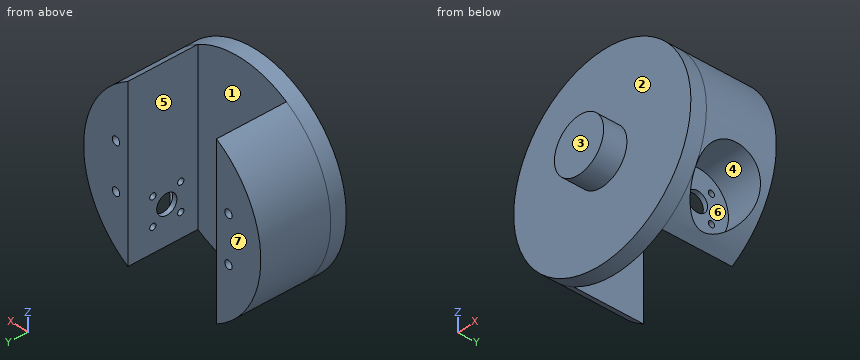
```python
from build123d import *

# Parameters (mm, degrees)
SKETCH1_R           = 17.5
BOSS_EXTRUDE1_DEPTH = 15
SKETCH2_R           = 63
BOSS_EXTRUDE2_DEPTH = 10
BOSS_EXTRUDE3_DEPTH = 45
SKETCH5_R           = 2.625
CUT_EXTRUDE1_DEPTH  = 6
SKETCH7_R           = 20
CUT_EXTRUDE2_DEPTH  = 28.5
SKETCH9_R           = 2
SKETCH9_R_2         = 6.5
CUT_EXTRUDE3_DEPTH  = 31.5


with BuildPart() as part:
    # Sketch1 → Boss-Extrude1 (new body)
    with BuildSketch(Plane(origin=(0, 0, 0), x_dir=(1, 0, 0), z_dir=(0, 1, 0))):
        with Locations(Location((0, 0, 0), (0, 0, 270))):
            Circle(SKETCH1_R)
    extrude(amount=BOSS_EXTRUDE1_DEPTH)

    # Sketch2 → Boss-Extrude2 (add)
    with BuildSketch(Plane(origin=(0, 15, 0), x_dir=(1, 0, 0), z_dir=(0, 1, 0))):
        with Locations(Location((0, 0, 0), (0, 0, 270))):
            Circle(SKETCH2_R)
    extrude(amount=BOSS_EXTRUDE2_DEPTH)

    # Sketch4 → Boss-Extrude3 (add)
    with BuildSketch(Plane(origin=(0, 25, 0), x_dir=(1, 0, 0), z_dir=(0, 1, 0))):
        with BuildLine():
            Line((-31.5, 44), (-31.5, 54.559600438))
            ThreePointArc((-31.5, 54.559600438), (-63, 0), (-31.5, -54.559600438))
            Line((-31.5, -54.559600438), (-31.5, -44))
            Line((-31.5, -44), (-31.5, 44))
        make_face()
        with BuildLine():
            Line((31.5, -44), (31.5, 44))
            Line((31.5, 44), (31.5, 54.559600438))
            ThreePointArc((31.5, 54.559600438), (63, 0), (31.5, -54.559600438))
            Line((31.5, -54.559600438), (31.5, -44))
        make_face()
    extrude(amount=BOSS_EXTRUDE3_DEPTH)

    # Sketch5 → Cut-Extrude1 (cut)
    with BuildSketch(Plane(origin=(0, 70, 0), x_dir=(1, 0, 0), z_dir=(0, 1, 0))):
        with Locations(Location((-40, 15, 0), (0, 0, 270))):
            Circle(SKETCH5_R)
        with Locations(Location((-40, -15, 0), (0, 0, 270))):
            Circle(SKETCH5_R)
        with Locations(Location((40, -15, 0), (0, 0, 90))):
            Circle(SKETCH5_R)
        with Locations(Location((40, 15, 0), (0, 0, 90))):
            Circle(SKETCH5_R)
    extrude(amount=-CUT_EXTRUDE1_DEPTH, mode=Mode.SUBTRACT)

    # Sketch7 → Cut-Extrude2 (cut)
    with BuildSketch(Plane(origin=(63, 0, 0), x_dir=(0, 0, -1), z_dir=(1, 0, 0))):
        with Locations((30, 45)):
            Circle(SKETCH7_R)
    extrude(amount=-CUT_EXTRUDE2_DEPTH, mode=Mode.SUBTRACT)

    # Sketch9 → Cut-Extrude3 (cut)
    with BuildSketch(Plane(origin=(63, 0, 0), x_dir=(0, 0, -1), z_dir=(1, 0, 0))):
        with Locations((21.019743879, 36.019743879)):
            Circle(SKETCH9_R)
        with Locations((21.019743879, 53.980256121)):
            Circle(SKETCH9_R)
        with Locations((38.980256121, 53.980256121)):
            Circle(SKETCH9_R)
        with Locations((38.980256121, 36.019743879)):
            Circle(SKETCH9_R)
        with Locations((30, 45)):
            Circle(SKETCH9_R_2)
    extrude(amount=-CUT_EXTRUDE3_DEPTH, mode=Mode.SUBTRACT)


solid = part.part
```
For this review, take the finished solid that the model builds, in its own axes (mm). Face numbers are marked on the shaded views. A direction names the side the tool comes from. Round coordinates to 2 decimals unless told otherwise and drop trailing zeros. Write each loop counter-clockwise with the first axis right and the second up, starting at its lowest first coordinate (ties: lowest second). Pieces come first, ordered by that corner, then holes. Notation, with made-up numbers: M 34.5,77 L 44.5,77 A23 ccw 44.5,115 Z; hole C 18,11.5 d5. An arc over 180 degrees is marked long. One line per item, written item: value. Start each with the question number.
(1) We need section B-B (y = 29). Give the boundary of the cut face in (x, z).
(2) We need section D-D (y = 45). Give the boundary of the cut face in (x, z).
(3) We need section A-A (z = -30). Give the boundary of the cut face in (x, y).
(4) We need section C-C (x = 0). Give the boundary of the cut face in (y, z), and give its area (4 significant figures).
(5) The part is to be moulded in two halves that separate along X. For the marked faces 5, 6 and 7, say which applies: released by +X, released by -X, zero draft, split by the parting line, or undercut.
(6) Machinability: for the marked faces 1, 2, 3 and 4, which of the approach directions +Z, -Z, +X, -X, +Y, -Y give a long, thin tool a straight path to every point of the face, cutting with its end or side? Answer none if there is none.
(7) Insertion check: pin 1 (10 mm diameter, centred on y = 41.5, z = 44, fed in from -X); pin 2 (1 mm diameter, centred on x = 16.5, z = -28, fed in from -Y); pin 3 (1.6 mm diameter, centred on x = 40.5, z = 14, fed in from +Y). Each pin has a flat end and moves straight along its axis. Give the tip position at first contact, or say it passes through.
(8) Wall thickness on line 1 (Z direction, x = 40, y = 68.45) (3 decimals); line 2 (X direction, y = 67.55, z = 15) (3 decimals); line 3 (Y direction, x = 27, z = 5.5): over which ranges is each line inside the solid? List them lowest first.
Result:
1. outline: M -31.5,-54.56 L -31.5,54.56 A63 ccw Z; M 31.5,-54.56 A63 ccw 46.96,-42 L 34.5,-42 L 34.5,-18 L 60.37,-18 A63 ccw 31.5,54.56 Z
2. outline: M -31.5,-54.56 L -31.5,54.56 A63 ccw Z; M 31.5,-54.56 A63 ccw 38.33,-50 L 34.5,-50 L 34.5,-36.5 L 31.5,-36.5 Z; M 31.5,-23.5 L 34.5,-23.5 L 34.5,-10 L 62.2,-10 A63 ccw 31.5,54.56 Z
3. outline: M -55.4,15 L 55.4,15 L 55.4,25 L 34.5,25 L 34.5,38.5 L 31.5,38.5 L 31.5,25 L -31.5,25 L -31.5,70 L -55.4,70 Z; M 31.5,51.5 L 34.5,51.5 L 34.5,65 L 55.4,65 L 55.4,70 L 31.5,70 Z
4. outline: M 0,-17.5 L 15,-17.5 L 15,-63 L 25,-63 L 25,63 L 15,63 L 15,17.5 L 0,17.5 Z
4. area: 1,785 mm²
5. face 5: undercut
5. face 6: released by +X
5. face 7: zero draft
6. face 1: +Z, -Z, +Y
6. face 2: -Y
6. face 3: +Z, -Z, +X, -X, -Y
6. face 4: +X
7. pin 1: x = -49.48
7. pin 2: y = 15
7. pin 3: y = 64
8. line 1: -48.672 to -17.625, -12.375 to 12.375, 17.625 to 48.672
8. line 2: -61.188 to -42.625, -37.375 to -31.5, 31.5 to 37.375, 42.625 to 61.188
8. line 3: 15 to 25
